from build123d import *

# Parameters (mm, degrees)
SKETCH_2_R          = 3.5
CUT_EXTRUDE_1_DEPTH = 24


with BuildPart() as part:
    # 草图1 → 旋转1 (revolve)
    with BuildSketch(Plane(origin=(0, 0, 0), x_dir=(1, 0, 0), z_dir=(0, 1, 0))):
        with BuildLine():
            Line((4.47238179, 5.664226859), (8.542255744, 7.893258215))
            ThreePointArc((8.542255744, 7.893258215), (9.014848357, 9.073438454), (7.947303741, 9.763741043))
            Line((7.947303741, 9.763741043), (0, 8.847027754))
            Line((0, 8.847027754), (0, 3.743540559))
            Line((0, 3.743540559), (0, -3.743540559))
            Line((0, -3.743540559), (0, -8.847027754))
            Line((0, -8.847027754), (7.310640748, -9.114898963))
            ThreePointArc((7.310640748, -9.114898963), (8.319210693, -8.350743764), (7.771541106, -7.210040242))
            Line((7.771541106, -7.210040242), (4.47238179, -5.664226859))
            ThreePointArc((4.47238179, -5.664226859), (7.21703989, 0), (4.47238179, 5.664226859))
        make_face()
    revolve(axis=Axis((0, 0, 7.015647414), (0, 0, -1)))

    # 草图2 → 切除-拉伸1 (cut)
    with BuildSketch(Plane.XY.offset(-9.763741043)):
        with Locations(Location((0, 0, 0), (0, 0, 180))):
            Circle(SKETCH_2_R)
    extrude(amount=CUT_EXTRUDE_1_DEPTH, mode=Mode.SUBTRACT)


solid = part.part
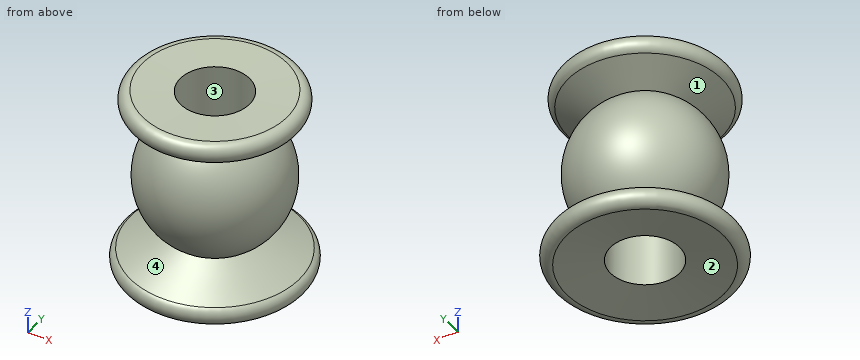
Here's how the part is built. I have some questions about the finished solid (model axes, mm). Face numbers are marked on the shaded views. A direction names the side the tool comes from. Coordinates: 2 decimals unless noted, no trailing zeros. Write each loop counter-clockwise with the first axis right and the second up, starting at its lowest first coordinate (ties: lowest second). Pieces come first, ordered by that corner, then holes.
Item 1: I want a section at D-D on x = 6.5. Count the separate pieces of the cut face and the enclosed holes in it, and give its area (3 significant figures).
Item 2: Will these pins go through, and if not, where does the flat tip stop? pin 1 (6 mm diameter, centred on y = 4, z = 5.5, fed in from -X); pin 2 (4 mm diameter, centred on x = -5, z = -4, fed in from +Y); pin 3 (1 mm diameter, centred on y = -3, z = -2, fed in from -X).
Item 3: On a 3-axis mill with a long thin cutter (end or side, diameter ignored), from which of +Z, -Z, +X, -X, +Y, -Y can I reach the whole of each face in a straight line? I mean the marked faces 1 and 2. Say none if no direction works.
Item 4: I want a section at C-C on z = 0. Write out the boundary of the cut face in (x, y), and give its area (3 significant figures).
Item 5: If we mould it in two halves opening along Y, with no side actions, what happens to the marked faces 3 and 4? For each: +Y half, -Y half, draft (parallel to the pull), parting line (faces both ways), or undercut.
Item 6: I want a section at A-A on y = 0. Write out the boundary of the cut face in (x, z).
Item 7: If I drill on line 1 (Z direction, x = -5, y = 2.5); line 2 (Z direction, x = 6.5, y = 0); line 3 (Y direction, x = -2.25, z = -6), over which ranges is the centre line in solid material (lowest first)?
Findings below:
1. separate pieces: 3
1. enclosed holes: 0
1. area: 82.5 mm2
2. pin 1: stops at x = -8.03
2. pin 2: stops at y = 5.72
2. pin 3: stops at x = -6.51
3. face 1: none
3. face 2: -Z
4. outline: circle Ø14.43 at (0, 0); hole circle Ø7 at (0, 0)
4. area: 125 mm2
5. face 3: undercut
5. face 4: parting line
6. outline: (-8.54, -7.89) arc R1 ccw to (-7.95, -9.76) - (-3.5, -9.25) - (-3.5, 8.98) - (-7.31, 9.11) arc R1 ccw to (-7.77, 7.21) - (-4.47, 5.66) arc R7.22 ccw to (-4.47, -5.66) - close; (3.5, -9.25) - (7.95, -9.76) arc R1 ccw to (8.54, -7.89) - (4.47, -5.66) arc R7.22 ccw to (4.47, 5.66) - (7.77, 7.21) arc R1 ccw to (7.31, 9.11) - (3.5, 8.98) - close
7. line 1: z = -9.49 to -6.28, -4.56 to 4.56, 6.19 to 9.05
7. line 2: z = -9.6 to -6.77, -3.14 to 3.14, 6.61 to 9.09
7. line 3: y = -4.56 to -2.68, 2.68 to 4.56
